Build history of the part. All positions in model axes, mm. A direction names the side the tool comes from. Give positions to 0.01 mm unless a question says otherwise; leave off trailing zeros. Order: outer loops, then holes, each group sorted by start corner. A loop starts at its lowest first (then second) coordinate and runs counter-clockwise, first axis right, second up. Notation, with made-up numbers: M 1.5,82 L 34.5,82 A19 ccw 34.5,93 Z; hole C 1.5,3 d7. An arc over 180 degrees is marked long. One line per item, written item: value.
from build123d import *

# Parameters (mm, degrees)
SKETCH1_W                                = 100
SKETCH1_H                                = 100
BOSS_EXTRUDE1_DEPTH                      = 15
BOSS_EXTRUDE2_DEPTH                      = 10
CBORE_FOR_M5_HEX_HEAD_BOLT2_D            = 5.8
CBORE_FOR_M5_HEX_HEAD_BOLT2_CBORE_D      = 10
CBORE_FOR_M5_HEX_HEAD_BOLT2_CBORE_DEPTH  = 5
FILLET1_R                                = 5
FILLET2_R                                = 10
SKETCH11_R                               = 32.5
BOSS_EXTRUDE3_DEPTH                      = 45
CBORE_FOR_M36_HEX_HEAD_BOLT2_D           = 20
CBORE_FOR_M36_HEX_HEAD_BOLT2_CBORE_D     = 40
CBORE_FOR_M36_HEX_HEAD_BOLT2_CBORE_DEPTH = 20


with BuildPart() as part:
    # Sketch1 → Boss-Extrude1 (new body)
    with BuildSketch(Plane(origin=(0, 0, 0), x_dir=(1, 0, 0), z_dir=(0, 1, 0))):
        with Locations((50, 50)):
            Rectangle(SKETCH1_W, SKETCH1_H)
    extrude(amount=BOSS_EXTRUDE1_DEPTH)

    # Sketch3 → Boss-Extrude2 (add)
    with BuildSketch(Plane(origin=(0, 15, 0), x_dir=(1, 0, 0), z_dir=(0, 1, 0))):
        with BuildLine():
            Line((37.5, 100), (37.5, 115.975098948))
            ThreePointArc((37.5, 115.975098948), (50, 128.475098948), (62.5, 115.975098948))
            Line((62.5, 115.975098948), (62.5, 100))
            Line((62.5, 100), (37.5, 100))
        make_face()
        with BuildLine():
            Line((62.5, 0), (62.5, -15))
            ThreePointArc((62.5, -15), (50, -27.5), (37.5, -15))
            Line((37.5, -15), (37.5, 0))
            Line((37.5, 0), (62.5, 0))
        make_face()
    extrude(amount=-BOSS_EXTRUDE2_DEPTH)

    # CBORE for M5 Hex Head Bolt2 (through all)
    with Locations(Plane(origin=(0, 15, 0), x_dir=(1, 0, 0), z_dir=(0, 1, 0))):
        with Locations((50, 115.975098948), (50, -15)):
            CounterBoreHole(CBORE_FOR_M5_HEX_HEAD_BOLT2_D / 2, CBORE_FOR_M5_HEX_HEAD_BOLT2_CBORE_D / 2, CBORE_FOR_M5_HEX_HEAD_BOLT2_CBORE_DEPTH)

    # Fillet1
    fillet1_edges = [part.edges().sort_by_distance(p)[0] for p in [
        (62.5, 10, -100),
        (37.5, 10, -100),
        (37.5, 10, 0),
        (62.5, 10, 0),
    ]]
    fillet(fillet1_edges, radius=FILLET1_R)

    # Fillet2
    fillet2_edges = [part.edges().sort_by_distance(p)[0] for p in [
        (0, 7.5, -100),
        (100, 7.5, -100),
        (100, 7.5, 0),
        (0, 7.5, 0),
    ]]
    fillet(fillet2_edges, radius=FILLET2_R)

    # Sketch11 → Boss-Extrude3 (add)
    with BuildSketch(Plane(origin=(0, 15, 0), x_dir=(1, 0, 0), z_dir=(0, 1, 0))):
        with Locations(Location((50, 50, 0), (0, 0, 90))):
            Circle(SKETCH11_R)
    extrude(amount=BOSS_EXTRUDE3_DEPTH)

    # CBORE for M36 Hex Head Bolt2 (through all)
    with Locations(Plane(origin=(0, 60, 0), x_dir=(1, 0, 0), z_dir=(0, 1, 0))):
        with Locations((50, 50)):
            CounterBoreHole(CBORE_FOR_M36_HEX_HEAD_BOLT2_D / 2, CBORE_FOR_M36_HEX_HEAD_BOLT2_CBORE_D / 2, CBORE_FOR_M36_HEX_HEAD_BOLT2_CBORE_DEPTH)


solid = part.part
1) Saw through at B-B, the plane x = 20. Write the cut outline in (y, z), then the cut area to 4 significant figures.
Check values:
outline: M 0,-100 L 15,-100 L 15,-62.5 L 60,-62.5 L 60,-37.5 L 15,-37.5 L 15,0 L 0,0 Z
area: 2,625 mm^2
2) Pin check, flat tips, straight feed: pin 1 (2 mm diameter, centred on x = 40.5, z = -86.5, fed in from +Y); pin 2 (9 mm diameter, centred on x = 50, z = 15, fed in from -Y); pin 3 (4.5 mm diameter, centred on x = 44, y = 10.5, fed in from +Z). Stop position of each tip, or through.
Check values:
pin 1: y = 15
pin 2: y = 5
pin 3: z = 26.92
3) Mould opens along Z. For faces 6 (the face through (47.32, 7.46, 16.11)), 7 (the face through (36, 9.93, -101.43)), 8 (the face through (37.5, 10, -110)) say: released by +Z, released by -Z, zero draft, split by the parting line, or undercut.
Check values:
face 6: undercut
face 7: released by -Z
face 8: zero draft
4) Saw through at A-A, the plane z = -50. Write the cut outline in (x, y), then the cut area to 4 significant figures.
Check values:
outline: M 0,0 L 40,0 L 40,40 L 30,40 L 30,60 L 17.5,60 L 17.5,15 L 0,15 Z; M 60,0 L 100,0 L 100,15 L 82.5,15 L 82.5,60 L 70,60 L 70,40 L 60,40 Z
area: 2,825 mm^2
5) Drill centre lines: probe 1 along Z at (x, y) = (50, 12); probe 2 along Z at (x, y) = (50, 7); probe 3 along X at (y, z) = (29, -50). Where is each one in solid material? Low to high. Write a range as from..to.
Check values:
probe 1: -128.48..-120.98, -110.98..-60, -40..10, 20..27.5
probe 2: -128.48..-118.88, -113.08..-60, -40..12.1, 17.9..27.5
probe 3: 17.5..40, 60..82.5
6) Tool access for faces 1 (the face through (37.5, 10, 10)), 2 (the face through (49, 4, 0)), 3 (the face through (41, 40, -55)), 4 (the face through (50, 5, 11)), 5 (the face through (62.5, 10, -111)): list every direction of +Z, -Z, +X, -X, +Y, -Y with a clear straight run to the whole face (end or side of a thin tool).
Check values:
face 1: +Z, -X, +Y, -Y
face 2: +Z, -Y
face 3: +Y
face 4: +Z, +X, -X, -Y
face 5: -Z, +X, +Y, -Y
7) Saw through at C-C, the plane y = 51. Write the cut outline in (x, z), then the cut area to 3 significant figures.
Check values:
outline: C 50,-50 d65; hole C 50,-50 d40
area: 2,060 mm^2
8) Saw through at D-D, the plane z = -25.5. Write the cut outline in (x, y), then the cut area to 3 significant figures.
Check values:
outline: M 0,0 L 100,0 L 100,15 L 71.35,15 L 71.35,60 L 28.65,60 L 28.65,15 L 0,15 Z
area: 3,420 mm^2
